Part print with two shaded views. Sizes in mm from the minimum x, y, z corner. A direction names the side the tool comes from. Round coordinates to 2 decimals unless told otherwise and drop trailing zeros. Order: outer loops, then holes, each group sorted by start corner. A loop starts at its lowest first (then second) coordinate and runs counter-clockwise, first axis right, second up. Notation, with made-up numbers: (-6, -33) -> (8, -33) arc R27 cw to (8, -6) -> close; hole circle Ø4 at (-40, -2.75). An arc over 180 degrees is marked (long way). Answer as a JSON object with one key per item and string values.
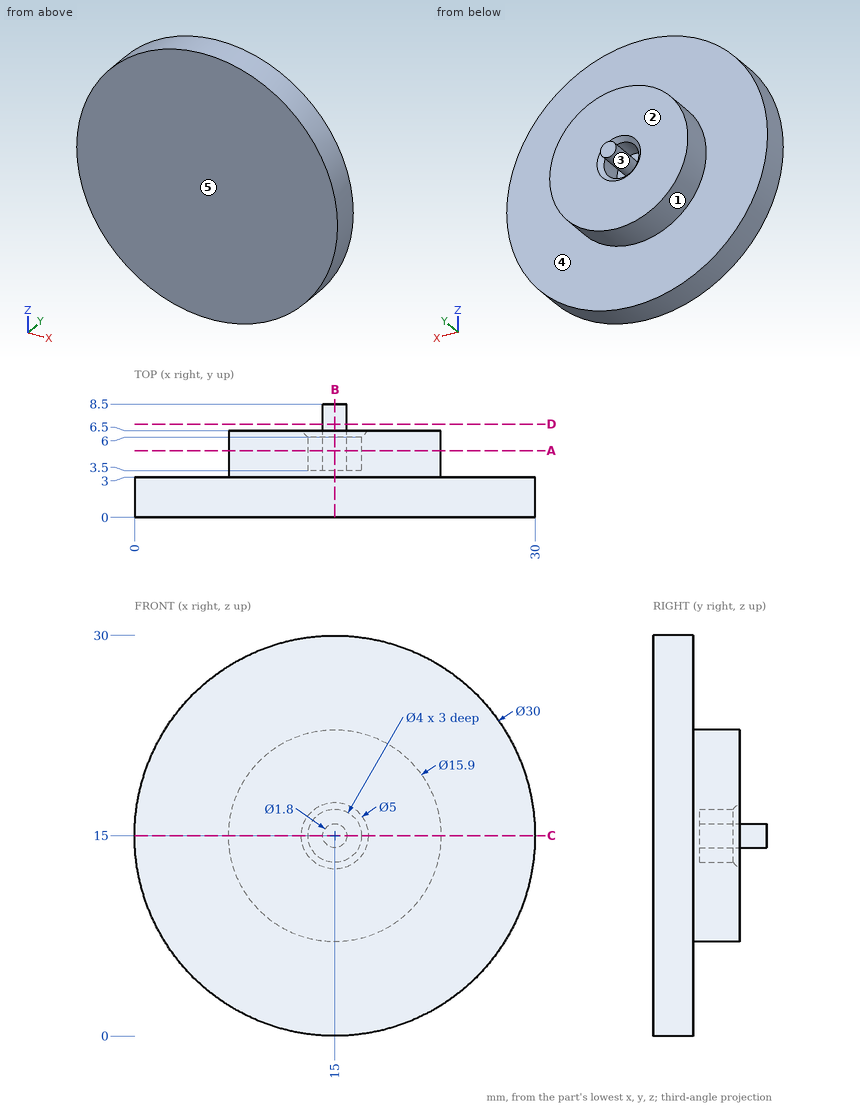
1) Probe L1, parallel to X at y = 4, z = 15; L2, parallel to Z at x = 14.25, y = 5.5. List the from-to ranges inside material, lowest first. Write a range as from..to.
Checked values:
{"L1": "x = 7.05..13, 14.1..15.9, 17..22.95", "L2": "z = 7.09..13.15, 14.5..15.5, 16.85..22.91"}
2) Cut at D-D, the plane y = 7. Give the cut face in (x, z), plus the area to 3 significant figures.
Checked values:
{"outline": "circle Ø1.8 at (15, 15)", "area": "2.54 mm²"}
3) Which spindle directions (+Z, -Z, +X, -X, +Y, -Y) get a long thin tool onto all of the face, cutting with end or side? Do the marked faces 4 and 5. Say none if no direction does.
Checked values:
{"face 4": "+Y", "face 5": "+Z, -Z, +X, -X, -Y"}
4) Cut at A-A, the plane y = 5. Give the cut face in (x, z).
Checked values:
{"outline": "circle Ø15.9 at (15, 15); circle Ø1.8 at (15, 15); hole circle Ø4 at (15, 15)"}
5) Cut at B-B, the plane x = 15. Give the cut face in (y, z), plus the area to 3 significant figures.
Checked values:
{"outline": "(0, 0) -> (3, 0) -> (3, 7.05) -> (6.5, 7.05) -> (6.5, 12.5) -> (6, 13) -> (3.5, 13) -> (3.5, 14.1) -> (8.5, 14.1) -> (8.5, 15.9) -> (3.5, 15.9) -> (3.5, 17) -> (6, 17) -> (6.5, 17.5) -> (6.5, 22.95) -> (3, 22.95) -> (3, 30) -> (0, 30) -> close", "area": "142 mm²"}
6) Cut at C-C, the plane z = 15. Give the cut face in (x, y).
Checked values:
{"outline": "(0, 0) -> (30, 0) -> (30, 3) -> (22.95, 3) -> (22.95, 6.5) -> (17.5, 6.5) -> (17, 6) -> (17, 3.5) -> (15.9, 3.5) -> (15.9, 8.5) -> (14.1, 8.5) -> (14.1, 3.5) -> (13, 3.5) -> (13, 6) -> (12.5, 6.5) -> (7.05, 6.5) -> (7.05, 3) -> (0, 3) -> close"}
7) Flat gauge pins, fed straight in: pin 1 Ø1 at (y, z) = (6, 19.5) entering from +X; pin 2 Ø2 at (x, z) = (7, 19.5) entering from +Y; pin 3 Ø2 at (y, z) = (3.5, 13) entering from -X. Where does each tip first touch, or does it go through?
Checked values:
{"pin 1": "stops at x = 21.87", "pin 2": "stops at y = 3", "pin 3": "stops at x = 0.04"}
8) Pull direction Z, two halves, no side cores. Call the marked faces 1, 2 and 3: pulls with the +Z half, pulls with the -Z half, needs draft (parallel to the pull), parting line crosses it, or undercut.
Checked values:
{"face 1": "parting line crosses it", "face 2": "needs draft", "face 3": "undercut"}
